Work out the finished part from the listing and answer in its coordinate system (mm). A direction names the side the tool comes from. Coordinates: 2 decimals unless noted, no trailing zeros. Order: outer loops, then holes, each group sorted by start corner. A loop starts at its lowest first (then second) coordinate and runs counter-clockwise, first axis right, second up.
1. The part is cut by section B-B, the plane y = 0. Give the vertices of the cut face in (x, z).
2. A tool of negligible diameter and unlimited length cuts with its end or side. For faces 5 (the flat face through (0, 0, 0)), 6 (the flat face through (20, -5, -2)), 7 (the flat face through (120, 6, -4)), from which of +Z, -Z, +X, -X, +Y, -Y can it reach the whole face along a straight path? Write none if from no direction.
3. The part is cut by section A-A, the plane z = 0. Give the vertices of the cut face in (x, y).
4. Flat-ended cylindrical pins translate along their axes: pin 1 Ø1 at (x, y) = (141.5, 4) entering from -Z; pin 2 Ø2.5 at (x, y) = (203, 4.5) entering from +Z; pin 3 Ø1.8 at (x, z) = (199, -1) entering from +Y. Find the tip coordinate at first contact, or state that the pin passes through.
5. The part is cut by section D-D, the plane x = 202. Give the vertices of the cut face in (y, z).
6. Determine the mould class of faces 1 (the cylindrical face through (182, 5, 0)), 2 (the flat face through (199, 3.2, 0)), 3 (the flat face through (215, 0, 0)), 4 (the cylindrical face through (168.165, -5.902, -3.763)) for opening direction Z: +Z half, -Z half, draft (parallel to the pull), parting line (faces both ways), or undercut.
7. Find the intervals of material crossed by probe 1 along Z at (x, y) = (110, 0.75); probe 2 along X at (y, z) = (3.75, 0.25); probe 3 along X at (y, z) = (3, 5.25), in increasing order.
8. The part is cut by section C-C, the plane x = 87. Give the vertices of the cut face in (y, z).
```python
from build123d import *

# Parameters (mm, degrees)
CHAMFER1_SIZE      = 1
CUT_EXTRUDE1_START = 3.2
CUT_EXTRUDE1_DEPTH = 10


# Read off the part's stored shape, not the designer's step: M10x1.0 Machine Threads Stud1
with BuildPart() as part:
    # Sketch1 → Revolve1 (revolve)
    with BuildSketch(Plane(origin=(0, 0, 0), x_dir=(1, 0, 0), z_dir=(0, 1, 0))):
        Polygon((0, 0), (0, 7), (20, 7), (20, 7.4), (120, 7.4), (120, 7), (215, 7), (215, 0), align=None)
    revolve(axis=Axis((215, 0, 0), (-1, 0, 0)))

    # M10x1.0 Machine Threads Stud1 outline → M10x1.0 Machine Threads Stud1 (revolve, cut)
    with BuildSketch(Plane.YX):
        Polygon((7, 20), (5, 20), (5, 0.5545), (4.4455, 0), (7, 0), align=None)
    revolve(axis=Axis((0, 0, 0), (1, 0, 0)), mode=Mode.SUBTRACT)

    # Chamfer1
    chamfer1_edges = [part.edges().sort_by_distance(p)[0] for p in [
        (20, 0, 7.4),
    ]]
    chamfer(chamfer1_edges, length=CHAMFER1_SIZE)

    # Sketch3 → Cut-Extrude1 (cut)
    with BuildSketch(Plane(origin=(0, 0, 0), x_dir=(1, 0, 0), z_dir=(0, 1, 0)).offset(CUT_EXTRUDE1_START)):
        with BuildLine():
            Line((245, -3), (185, -3))
            ThreePointArc((185, -3), (182, 0), (185, 3))
            Line((185, 3), (245, 3))
            Line((245, 3), (245, -3))
        make_face()
    extrude(amount=CUT_EXTRUDE1_DEPTH, mode=Mode.SUBTRACT)


solid = part.part
```
Geometry says:
1. outline: (0, -4.45) - (0.55, -5) - (20, -5) - (20, -6.4) - (21, -7.4) - (120, -7.4) - (120, -7) - (215, -7) - (215, 7) - (120, 7) - (120, 7.4) - (21, 7.4) - (20, 6.4) - (20, 5) - (0.55, 5) - (0, 4.45) - close
2. face 5: +Z, -Z, -X, +Y, -Y
2. face 6: -X
2. face 7: +X
3. outline: (0, -4.45) - (0.55, -5) - (20, -5) - (20, -6.4) - (21, -7.4) - (120, -7.4) - (120, -7) - (215, -7) - (215, 3.2) - (182, 3.2) - (182, 7) - (120, 7) - (120, 7.4) - (21, 7.4) - (20, 6.4) - (20, 5) - (0.55, 5) - (0, 4.45) - close
4. pin 1: stops at z = -6.06
4. pin 2: stops at z = 6.2
4. pin 3: stops at y = 3.2
5. outline: (3.2, -3) - (3.2, 3) - (6.32, 3) arc R7 ccw (long way) to (6.32, -3) - close
6. face 1: undercut
6. face 2: undercut
6. face 3: draft
6. face 4: parting line
7. probe 1: z = -7.36 to 7.36
7. probe 2: x = 0 to 182.01
7. probe 3: x = 20 to 215
8. outline: circle Ø14.8 at (0, 0)
